from build123d import *

# Parameters (mm, degrees)
SKETCH1_W           = 55
SKETCH1_H           = 5
SKETCH1_W_2         = 4.5
BOSS_EXTRUDE2_DEPTH = 20
SKETCH2_W           = 8
SKETCH2_H           = 8
BOSS_EXTRUDE3_DEPTH = 35
FILLET1_R           = 1
BOSS_EXTRUDE4_DEPTH = 4


with BuildPart() as part:
    # Sketch1 → Boss-Extrude2 (new body)
    with BuildSketch(Plane.XY):
        Rectangle(SKETCH1_W, SKETCH1_H)
        with Locations((-6.65, -5)):
            Rectangle(SKETCH1_W_2, SKETCH1_H)
        with Locations((6.65, -5)):
            Rectangle(SKETCH1_W_2, SKETCH1_H)
    extrude(amount=BOSS_EXTRUDE2_DEPTH)

    # Sketch2 → Boss-Extrude3 (add)
    with BuildSketch(Plane(origin=(0, 2.5, 0), x_dir=(1, 0, 0), z_dir=(0, 1, 0))):
        with Locations((23.5, -10)):
            Rectangle(SKETCH2_W, SKETCH2_H)
        with Locations((-23.5, -10)):
            Rectangle(SKETCH2_W, SKETCH2_H)
    extrude(amount=BOSS_EXTRUDE3_DEPTH)

    # Fillet1
    fillet1_edges = [part.edges().sort_by_distance(p)[0] for p in [
        (0, 2.5, 20),
        (0, 2.5, 0),
        (8.9, -7.5, 10),
        (4.4, -7.5, 10),
        (-4.4, -7.5, 10),
        (-8.9, -7.5, 10),
        (-27.5, 2.5, 17),
        (27.5, 2.5, 17),
        (-27.5, 2.5, 3),
        (27.5, 2.5, 3),
    ]]
    fillet(fillet1_edges, radius=FILLET1_R)

    # Sketch9 → Boss-Extrude4 (add, symmetric)
    with BuildSketch(Plane.XY.offset(10)):
        with BuildLine():
            Line((-19.5, 8.405065213), (-19.5, 2.5))
            Line((-19.5, 2.5), (-11.364093889, 2.5))
            ThreePointArc((-11.364093889, 2.5), (-16.092079197, 4.543150534), (-19.5, 8.405065213))
        make_face()
    boss_extrude4 = extrude(amount=BOSS_EXTRUDE4_DEPTH, both=True)

    # Mirror1: Boss-Extrude4 across plane
    add(boss_extrude4.mirror(Plane(origin=(0, 0, 0), x_dir=(0, 0, 1), z_dir=(1, 0, 0))))


solid = part.part
Work out the finished part from the listing and answer in its coordinate system (mm). A direction names the side the tool comes from. Give positions to 0.01 mm unless a question says otherwise; leave off trailing zeros. Order: outer loops, then holes, each group sorted by start corner. A loop starts at its lowest first (then second) coordinate and runs counter-clockwise, first axis right, second up. Notation, with made-up numbers: (60.5, 44) -> (80.5, 44) arc R22 ccw to (80.5, 83) -> close; hole circle Ø3 at (9.5, 79). An arc over 180 degrees is marked (long way). Answer as a JSON object with one key per item and string values. Group by question number.
1. Section D-D on z = 10.25 is taken. Determine the outline of the cut face in (x, y).
2. The mould has two halves that part along X. Classify faces 1 (the flat face through (0, -1, 20)), 2 (the flat face through (27.5, 13, 10)), 3 (the cylindrical face through (-16.03, 4.5, 10.06)): released by +X, released by -X, zero draft, split by the parting line, or undercut.
3. Section B-B on z = 2.5 is taken. Determine the outline of the cut face in (x, y).
4. Consider line 1 along X through (y, z) = (17.5, 9); line 2 along Y through (x, z) = (-21, 6.5); line 3 along Y through (x, z) = (24.5, 5). Determine where each line is inside the solid, lowest interval first. Write a range as [from, to].
5. A tool of negligible diameter and unlimited length cuts with its end or side. For faces 4 (the flat face through (8.9, -5, 10)), 5 (the cylindrical face through (16.03, 4.5, 10.06)), 6 (the flat face through (4.4, -5, 10)), 7 (the flat face through (-18, -2.5, 10)), from which of +Z, -Z, +X, -X, +Y, -Y can it reach the whole face along a straight path? Write none if from no direction.
6. Section C-C on x = 2.5 is taken. Determine the outline of the cut face in (y, z), plus the area to 3 significant figures.
7. Section A-A on y = 29.5 is taken. Determine the outline of the cut face in (x, z).
8. Flat-ended cylindrical pins translate along their axes: pin 1 Ø5 at (x, y) = (-20.5, 19) entering from +Z; pin 2 Ø1.5 at (x, z) = (20.5, 4.5) entering from +Y; pin 3 Ø1.2 at (y, z) = (-4.5, 12.5) entering from +X; pin 4 Ø5 at (x, y) = (16.5, 25) entering from +Z. Find the tip coordinate at first contact, or state that the pin passes through.
Result sheet:
{
 "1": {"outline": "(-27.5, -2.5) -> (-8.9, -2.5) -> (-8.9, -6.5) arc R1 ccw to (-7.9, -7.5) -> (-5.4, -7.5) arc R1 ccw to (-4.4, -6.5) -> (-4.4, -2.5) -> (4.4, -2.5) -> (4.4, -6.5) arc R1 ccw to (5.4, -7.5) -> (7.9, -7.5) arc R1 ccw to (8.9, -6.5) -> (8.9, -2.5) -> (27.5, -2.5) -> (27.5, 37.5) -> (19.5, 37.5) -> (19.5, 8.41) arc R11.8 cw to (11.36, 2.5) -> (-11.36, 2.5) arc R11.8 cw to (-19.5, 8.41) -> (-19.5, 37.5) -> (-27.5, 37.5) -> close"},
 "2": {"face 1": "zero draft", "face 2": "released by +X", "face 3": "undercut"},
 "3": {"outline": "(-27.5, -2.5) -> (-8.9, -2.5) -> (-8.9, -6.5) arc R1 ccw to (-7.9, -7.5) -> (-5.4, -7.5) arc R1 ccw to (-4.4, -6.5) -> (-4.4, -2.5) -> (4.4, -2.5) -> (4.4, -6.5) arc R1 ccw to (5.4, -7.5) -> (7.9, -7.5) arc R1 ccw to (8.9, -6.5) -> (8.9, -2.5) -> (27.5, -2.5) -> (27.5, 1.5) arc R1 ccw to (26.5, 2.5) -> (-26.5, 2.5) arc R1 ccw to (-27.5, 1.5) -> close"},
 "4": {"line 1": "x = [-27.5, -19.5], [19.5, 27.5]", "line 2": "y = [-2.5, 37.5]", "line 3": "y = [-2.5, 2.5]"},
 "5": {"face 4": "+Z, -Z, +X, -Y", "face 5": "+Z, -Z, +Y", "face 6": "+Z, -Z, -Y", "face 7": "+Z, -Z, -X, -Y"},
 "6": {"outline": "(-2.5, 0) -> (1.5, 0) arc R1 ccw to (2.5, 1) -> (2.5, 19) arc R1 ccw to (1.5, 20) -> (-2.5, 20) -> close", "area": "99.6 mm^2"},
 "7": {"outline": "(-27.5, 6) -> (-19.5, 6) -> (-19.5, 14) -> (-27.5, 14) -> close; (19.5, 6) -> (27.5, 6) -> (27.5, 14) -> (19.5, 14) -> close"},
 "8": {"pin 1": "stops at z = 14", "pin 2": "stops at y = 2.5", "pin 3": "stops at x = 8.9", "pin 4": "passes through"}
}
